Verification items for the finished model (mm, model axes). A direction names the side the tool comes from. Give positions to 0.01 mm unless a question says otherwise; leave off trailing zeros. Order: outer loops, then holes, each group sorted by start corner. A loop starts at its lowest first (then second) coordinate and runs counter-clockwise, first axis right, second up.
(1) Gauge pin test, flat ends, axial feed: pin 1 (0.8 mm diameter, centred on x = 0.5, y = -0.5, fed in from -Z); pin 2 (1.5 mm diameter, centred on y = 1.5, z = 8.5, fed in from -X); pin 3 (1.5 mm diameter, centred on y = 0.5, z = 12.5, fed in from +X). Record the tip position at first contact, or that the pin passes through.
(2) Access from +Z, -Z, +X, -X, +Y, -Y to the whole of each face (thin tool, end or side, straight path). Record for faces 1 (the face through (0, 1.33, 1)), 2 (the face through (-1.43, -0.45, 15.32)).
(3) Sectioned sample at B-B on z = 23.5. Record the cut outline in (x, y), plus the area to 3 significant figures.
(4) Mould release check, pull along Y, two halves, no side actions. Record for faces 3 (the face through (-1.157, 0.656, 0.986)), 4 (the face through (0, 0, 2)), 5 (the face through (0, 0, 28.5)), 6 (the face through (0, -2, 1)): pulls with the +Y half, pulls with the -Y half, needs draft (parallel to the pull), parting line crosses it, or undercut.
(5) Sectioned sample at A-A on x = 0. Record the cut outline in (y, z).
(6) Scan lines: L1, parallel to X at y = 0.7, z = 14.75; L2, parallel to Z at x = -0.15, y = 0.25; L3, parallel to Z at x = -1.1, y = -1.3. Record each from-to range of solid material in increasing order.
```python
from build123d import *

# Parameters (mm, degrees)
ESQUISSE1_R             = 2
BASE_EXTRUSION_DEPTH    = 2.5
ESQUISSE2_R             = 1.5
BOSS_EXTRU_1_DEPTH      = 26
CONG_1_R                = 0.3
ENL_V_MAT_EXTRU_1_DEPTH = 2


with BuildPart() as part:
    # Esquisse1 → Base-Extrusion (new body)
    with BuildSketch(Plane.XY):
        Circle(ESQUISSE1_R)
    extrude(amount=BASE_EXTRUSION_DEPTH)

    # Esquisse2 → Boss.-Extru.1 (add)
    with BuildSketch(Plane.XY.offset(2.5)):
        with Locations(Location((0, 0, 0), (0, 0, 180))):
            Circle(ESQUISSE2_R)
    extrude(amount=BOSS_EXTRU_1_DEPTH)

    # Congé1
    cong_1_edges = [part.edges().sort_by_distance(p)[0] for p in [
        (-2, 0, 0),
    ]]
    fillet(cong_1_edges, radius=CONG_1_R)

    # Esquisse3 → Enlèv. mat.-Extru.1 (cut)
    with BuildSketch(Plane(origin=(0, 0, 0), x_dir=(-1, 0, 0), z_dir=(0, 0, -1))):
        Polygon((1.535751716, 0), (0.767875858, 1.33), (-0.767875858, 1.33), (-1.535751716, 0), (-0.767875858, -1.33), (0.767875858, -1.33), align=None)
    extrude(amount=-ENL_V_MAT_EXTRU_1_DEPTH, mode=Mode.SUBTRACT)


solid = part.part
```
Ans:
1. pin 1: stops at z = 2
1. pin 2: stops at x = -1.3
1. pin 3: stops at x = 1.5
2. face 1: -Z
2. face 2: +Z
3. outline: circle Ø3 at (0, 0)
3. area: 7.07 mm2
4. face 3: undercut
4. face 4: undercut
4. face 5: needs draft
4. face 6: parting line crosses it
5. outline: (-2, 0.3) arc R0.3 ccw to (-1.7, 0) - (-1.33, 0) - (-1.33, 2) - (1.33, 2) - (1.33, 0) - (1.7, 0) arc R0.3 ccw to (2, 0.3) - (2, 2.5) - (1.5, 2.5) - (1.5, 28.5) - (-1.5, 28.5) - (-1.5, 2.5) - (-2, 2.5) - close
6. L1: x = -1.33 to 1.33
6. L2: z = 2 to 28.5
6. L3: z = 0 to 2.5
